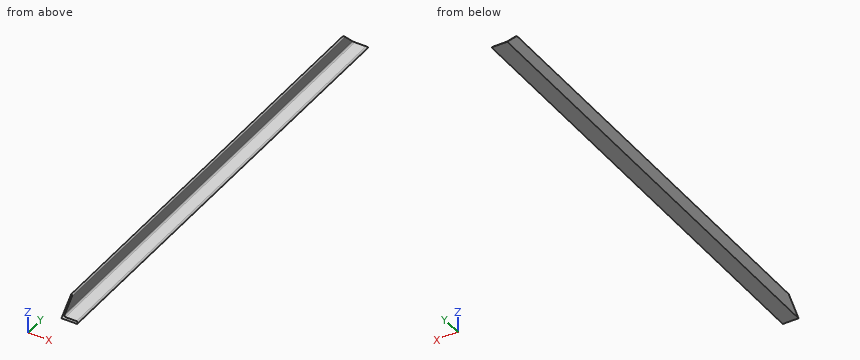
```python
from build123d import *

# Parameters (mm, degrees)
F2_DEPTH = 1524
F4_DEPTH = 50.8


# Not quite as in the source:
# - a variable given as a bare number and used for a length is read in inches; the dataset says mm whatever the document's units were


with BuildPart() as f2:
    # F1 (on Front) → F2 (new body)
    with BuildSketch(Plane.XZ):
        with BuildLine():
            ThreePointArc((4.7625, -4.7625), (3.3675960454, -1.3949039546), (0, 0))
            Line((0, 0), (0, -50.8))
            Line((0, -50.8), (50.8, -50.8))
            ThreePointArc((50.8, -50.8), (49.4050960454, -47.4324039546), (46.0375, -46.0375))
            Line((46.0375, -46.0375), (9.525, -46.0375))
            ThreePointArc((9.525, -46.0375), (6.1574039546, -44.6425960454), (4.7625, -41.275))
            Line((4.7625, -41.275), (4.7625, -4.7625))
        make_face()
    extrude(amount=-F2_DEPTH)

    # F3 (on face) → F4 (cut)
    with BuildSketch(Plane(origin=(0, 0, 0), x_dir=(0, -1, 0), z_dir=(-1, 0, 0))):
        Polygon((-50.8, 0), (0, -50.8), (0, 0), align=None)
        Polygon((-1524, 0), (-1524, -50.8), (-1473.2, 0), align=None)
    extrude(amount=-F4_DEPTH, mode=Mode.SUBTRACT)


solid = f2.part
```
Build history of the part. All positions in model axes, mm. Coordinates: 2 decimals unless noted, no trailing zeros. Order: outer loops, then holes, each group sorted by start corner. A loop starts at its lowest first (then second) coordinate and runs counter-clockwise, first axis right, second up.
Item 1: Saw through at B-B on z = -19.5. List the corners of the cut face in (x, y).
Filled in:
outline: (0, 31.3) - (4.76, 31.3) - (4.76, 1492.7) - (0, 1492.7) - close
Item 2: Drop flat-ended pins along their axis: pin 1 Ø12 at (y, z) = (1356.5, -24.5) entering from +X; pin 2 Ø8 at (x, z) = (42.5, -40.5) entering from -Y; pin 3 Ø1.5 at (y, z) = (838.5, -14.5) entering from -X. Give the stop position or say it passes through.
Filled in:
pin 1: stops at x = 4.76
pin 2: passes through
pin 3: stops at x = 0
Item 3: Saw through at A-A on y = 343.5. List the corners of the cut face in (x, z) (1 decimal).
Filled in:
outline: (0, -50.8) - (50.8, -50.8) arc R4.8 ccw to (46, -46) - (9.5, -46) arc R4.8 cw to (4.8, -41.3) - (4.8, -4.8) arc R4.8 ccw to (0, 0) - close
Item 4: Saw through at C-C on x = 31. List the corners of the cut face in (y, z), then the cut area to 3 significant figures.
Filled in:
outline: (0, -50.8) - (1524, -50.8) - (1519.24, -46.04) - (4.76, -46.04) - close
area: 7,240 mm2
Item 5: Drill centre lines: L1, parallel to X at y = 485.5, z = -37.5; L2, parallel to Z at x = 25, y = 906; L3, parallel to X at y = 961.5, z = -49. Where is each one in solid material? Low to high.
Filled in:
L1: x = 0 to 4.76
L2: z = -50.8 to -46.04
L3: x = 0 to 50.45
